For this review, use the dimensioned drawing (mm, ordinates from the lowest corner) and the shaded views. Coordinates: 2 decimals unless noted, no trailing zeros. Write each loop counter-clockwise with the first axis right and the second up, starting at its lowest first coordinate (ties: lowest second). Pieces come first, ordered by that corner, then holes. Notation, with made-up numbers: (-39, 37) -> (6, 37) arc R19 ccw to (6, 62) -> close; hole circle Ø8 at (81.25, 51). An arc over 180 degrees is marked (long way). Return JSON: item names as keys, results as strings. Group by question number.
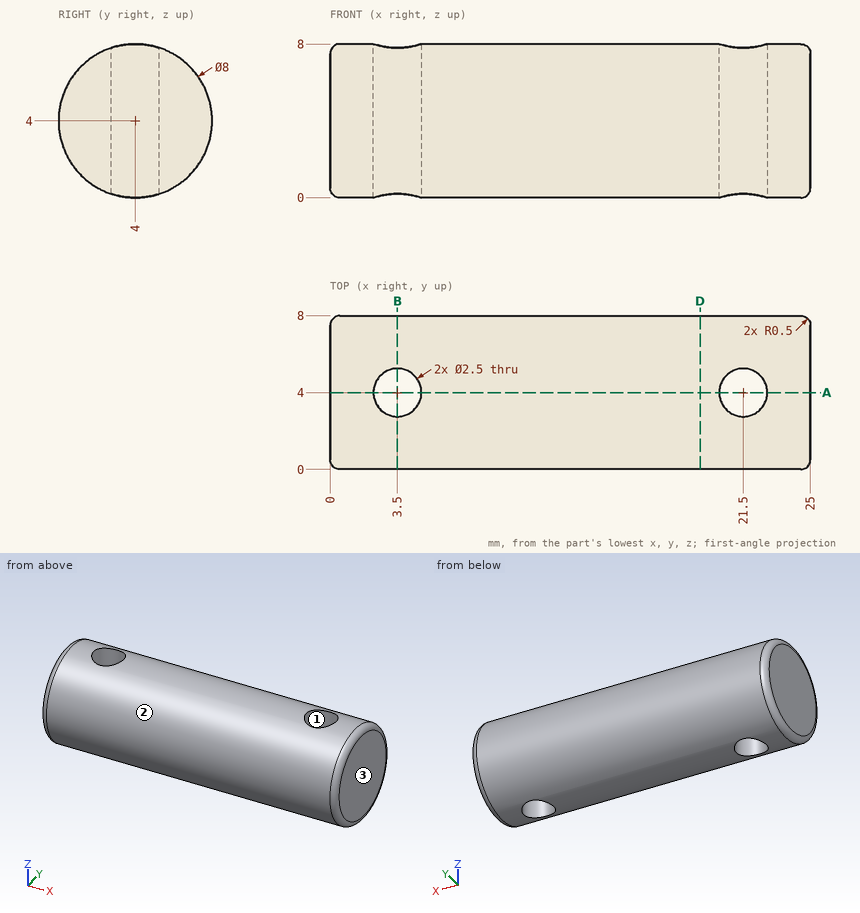
Q1. The part is to be moulded in two halves that separate along Y. For the marked faces 1, 2 and 3, say which applies: +Y half, -Y half, draft (parallel to the pull), parting line (faces both ways), or undercut.
Q2. Wall thickness on L1, parallel to Y at x = 3.5, z = 4.5; L2, parallel to X at y = 4.5, z = 2.5; L3, parallel to Y at x = 3.5, z = 6.25: over which ranges is each line inside the solid? List them lowest first.
Q3. We need section D-D on x = 19.25. Write out the cut boundary in (y, z).
Q4. We need section A-A on y = 4. State how many separate pieces and enclosed holes the cut face has, plus the area to 3 significant figures.
Q5. For P1, Ø1, axis at x = 15, z = 1, coming from the +Y side; P2, Ø2, axis at x = 21.5, z = 1.5, coming from the +Y side, all flat-tipped, find the tip position at first contact; note any pin that passes through.
Q6. We need section B-B on x = 3.5. Write out the cut boundary in (y, z).
Findings below:
{
 "1": {"face 1": "undercut", "face 2": "parting line", "face 3": "draft"},
 "2": {"L1": "y = 0.03 to 2.75, 5.25 to 7.97", "L2": "x = 0 to 2.35, 4.65 to 20.35, 22.65 to 25", "L3": "y = 0.69 to 2.75, 5.25 to 7.31"},
 "3": {"outline": "circle Ø8 at (4, 4)"},
 "4": {"separate pieces": "3", "enclosed holes": "0", "area": "160 mm^2"},
 "5": {"P1": "stops at y = 7.12", "P2": "stops at y = 7.71"},
 "6": {"outline": "(2.75, 0.2) -> (2.75, 7.8) arc R4 ccw to start; (5.25, 0.2) arc R4 ccw to (5.25, 7.8) -> close"}
}
